from build123d import *

# Parameters (mm, degrees)
SKETCH3_R           = 24.5
BOSS_EXTRUDE1_DEPTH = 10
SKETCH4_R           = 15.5
BOSS_EXTRUDE3_DEPTH = 4


with BuildPart() as part:
    # Sketch1 → Revolve1 (revolve)
    with BuildSketch(Plane.XY):
        Polygon((-50.994307358, 48.889927559), (-50.994307358, -61.110072441), (-36.994307358, -61.110072441), (-37.994307358, 48.889927559), align=None)
    revolve(axis=Axis((-37.994307358, 48.889927559, 0), (0.009090533456791595, -0.9999586802470746, 0)))

    # Sketch3 → Boss-Extrude1 (add)
    with BuildSketch(Plane(origin=(0, 48.544964037, 0), x_dir=(1, 0, 0), z_dir=(0, 1, 0))):
        with Locations(Location((-37.994307358, 0, 0), (0, 0, 270))):
            Circle(SKETCH3_R)
    extrude(amount=BOSS_EXTRUDE1_DEPTH)

    # Sketch4 → Boss-Extrude3 (add)
    with BuildSketch(Plane(origin=(0, -16.455035963, 0), x_dir=(1, 0, 0), z_dir=(0, 1, 0))):
        with Locations(Location((-37.494307358, 0, 0), (0, 0, 270))):
            Circle(SKETCH4_R)
    extrude(amount=BOSS_EXTRUDE3_DEPTH)


solid = part.part
Design review of the part built by this model. Coordinates are the model's own, in mm. A direction names the side the tool comes from. Give positions to 0.01 mm unless a question says otherwise; leave off trailing zeros. Write each loop counter-clockwise with the first axis right and the second up, starting at its lowest first coordinate (ties: lowest second). Pieces come first, ordered by that corner, then holes. Notation, with made-up numbers: M 9.25,88 L 66.25,88 A15 cw 66.25,94 Z; hole C 41,36 d5. An arc over 180 degrees is marked long. Return JSON: item names as keys, results as strings. Group by question number.
Item 1: Tool access review of faces 1 (the flat face through (-38, 58.545, 0)), 2 (the cylindrical face through (-46.926, -14.483, -12.3)), 3 (the flat face through (-51.2, -12.455, -0.1)), 4 (the cylindrical face through (-30.64, 53.47, 23.37)): name each direction out of +Z, -Z, +X, -X, +Y, -Y from which nothing blocks a thin tool from reaching the whole face with its end or side.
Item 2: Wall thickness on line 1 along Y through (x, z) = (-35, 15); line 2 along Y through (x, z) = (-43, 19); line 3 along Y through (x, z) = (-27.5, 2.5): over which ranges is each line inside the solid? List them lowest first.
Item 3: Take a section at A-A (x = -19). Give the boundary of the cut face in (y, z).
Item 4: Clearance check with flat-ended pins moving along their axes: pin 1 Ø4 at (y, z) = (-25, -5) entering from +X; pin 2 Ø10 at (y, z) = (-3.5, 5.5) entering from -X (3 decimals); pin 3 Ø6 at (y, z) = (-15.5, 4) entering from -X. State where each tip first meets the part, or that it passes through.
Return value:
{
 "1": {"face 1": "+Z, -Z, +X, -X, +Y", "face 2": "-Y", "face 3": "none", "face 4": "+Y, -Y"},
 "2": {"line 1": "y = -16.46 to -12.46, 48.54 to 58.54", "line 2": "y = 48.54 to 58.54", "line 3": "y = -60.93 to 58.54"},
 "3": {"outline": "M 48.54,-15.47 L 58.54,-15.47 L 58.54,15.47 L 48.54,15.47 Z"},
 "4": {"pin 1": "stops at x = -23.98", "pin 2": "stops at x = -50.985", "pin 3": "stops at x = -52.96"}
}
